Design review of the part built by this model. Coordinates are the model's own, in mm. Give positions to 0.01 mm unless a question says otherwise; leave off trailing zeros. Loops run counter-clockwise (first coordinate to the right, second up) from the corner with the lowest first, then second, coordinate; pieces in that order, holes last. Notation, with made-up numbers: (16, 53) -> (38, 53) arc R11 cw to (38, 57) -> close; hole circle Ø7 at (75.5, -27.75). An arc over 180 degrees is marked (long way). Use a Markdown table: item, result. Add a question column.
1. Add section D-D (y = 65.5). State the section outline as (x, z) points.
2. Draft analysis for pull direction X (two halves, no side actions). For faces 1 (the cylindrical face through (-15.46, 27.95, 0.99)), 2 (the cylindrical face through (-44.693, 9.549, 0.986)), 3 (the cylindrical face through (27, 96, 1)), state which applies: pulls with the +X half, pulls with the -X half, needs draft (parallel to the pull), parting line crosses it, or undercut.
3. Add section A-A (z = 0.55). State the section outline as (x, y) points, and give its area (3 significant figures).
4. Add section B-B (x = -28). State the section outline as (y, z) points.
5. Add section C-C (y = 27.5). State the section outline as (x, z) points, and give its area (3 significant figures).
6. For pin 1 Ø1 at (y, z) = (74, 1) entering from +X; pin 2 Ø0.6 at (x, z) = (2, 1) entering from +Y, all flat-tipped, find the tip position at first contact; note any pin that passes through.
7. To check wall thickness, follow line 1 (X direction, y = 81.5, z = 0.6); line 2 (Y direction, x = -25, z = 0.7); line 3 (X direction, y = 86, z = 1.65). State the ranges of each line that lie inside material, in increasing order.
```python
from build123d import *

# Parameters (mm, degrees)
IZIM2_R                     = 10
Y_KSEKLIK_EKSTR_ZYON1_DEPTH = 2


with BuildPart() as part:
    # Çizim2 → Yükseklik-Ekstrüzyon1 (new body)
    with BuildSketch(Plane.XY):
        with BuildLine():
            Line((-15, 100), (-15, 50))
            Line((-15, 50), (15, 50))
            Line((15, 50), (15, 100))
            ThreePointArc((15, 100), (27.116614772, 95.911871243), (34.279801416, 85.318764647))
            Line((34.279801416, 85.318764647), (49.09975177, 31.59845198))
            ThreePointArc((49.09975177, 31.59845198), (44.889839054, 9.804227706), (25, -0.050003828))
            Line((25, -0.050003828), (-25, -0.050003828))
            ThreePointArc((-25, -0.050003828), (-44.889839054, 9.804227706), (-49.09975177, 31.59845198))
            Line((-49.09975177, 31.59845198), (-34.279801416, 85.318764647))
            ThreePointArc((-34.279801416, 85.318764647), (-27.116614772, 95.911871243), (-15, 100))
        make_face()
        with Locations((-25, 24.949996172)):
            Circle(IZIM2_R, mode=Mode.SUBTRACT)
        with Locations((25, 24.949996172)):
            Circle(IZIM2_R, mode=Mode.SUBTRACT)
    extrude(amount=Y_KSEKLIK_EKSTR_ZYON1_DEPTH)


solid = part.part
```
Taken from the geometry:
| question | item | result |
|---|---|---|
| 1 | outline | (-39.75, 0) -> (-15, 0) -> (-15, 2) -> (-39.75, 2) -> close; (15, 0) -> (39.75, 0) -> (39.75, 2) -> (15, 2) -> close |
| 2 | face 1 | undercut |
| 2 | face 2 | pulls with the -X half |
| 2 | face 3 | pulls with the +X half |
| 3 | outline | (-49.1, 31.6) arc R25 ccw to (-25, -0.05) -> (25, -0.05) arc R25 ccw to (49.1, 31.6) -> (34.28, 85.32) arc R20 ccw to (15, 100) -> (15, 50) -> (-15, 50) -> (-15, 100) arc R20 ccw to (-34.28, 85.32) -> close; hole circle Ø20 at (-25, 24.95); hole circle Ø20 at (25, 24.95) |
| 3 | area | 6,100 mm^2 |
| 4 | outline | (0.13, 0) -> (15.41, 0) -> (15.41, 2) -> (0.13, 2) -> close; (34.49, 0) -> (95.2, 0) -> (95.2, 2) -> (34.49, 2) -> close |
| 5 | outline | (-49.87, 0) -> (-34.67, 0) -> (-34.67, 2) -> (-49.87, 2) -> close; (-15.33, 0) -> (15.33, 0) -> (15.33, 2) -> (-15.33, 2) -> close; (34.67, 0) -> (49.87, 0) -> (49.87, 2) -> (34.67, 2) -> close |
| 5 | area | 122 mm^2 |
| 6 | pin 1 | stops at x = 37.54 |
| 6 | pin 2 | stops at y = 50 |
| 7 | line 1 | x = -35.33 to -15, 15 to 35.33 |
| 7 | line 2 | y = -0.05 to 14.95, 34.95 to 97.32 |
| 7 | line 3 | x = -34.08 to -15, 15 to 34.08 |
